```python
from build123d import *

# Parameters (mm, degrees)
BASE_FLANGE1_DEPTH = 6.35
SKETCH8_R          = 3.4
CUT_EXTRUDE1_DEPTH = 183.851914127
SKETCH9_R          = 34
CUT_EXTRUDE2_DEPTH = 183.851914127
SKETCH10_R         = 2.75
CUT_EXTRUDE3_DEPTH = 183.851914127


# Sheet-metal steps are written as plain solids
with BuildPart() as part:
    # Sketch2 → Base-Flange1 (new body)
    with BuildSketch(Plane(origin=(0, 0, 0), x_dir=(1, 0, 0), z_dir=(0, 1, 0))):
        with BuildLine():
            Line((0, 0), (50.76093065, 0))
            Line((50.76093065, 0), (107.880465325, 57.119534675))
            ThreePointArc((107.880465325, 57.119534675), (111.537953618, 118.761570635), (50.76093065, 129.682710556))
            Line((50.76093065, 129.682710556), (0, 90))
            Line((0, 90), (0, 0))
        make_face()
    extrude(amount=-BASE_FLANGE1_DEPTH)

    # Sketch8 → Cut-Extrude1 (cut, through all)
    with BuildSketch(Plane(origin=(0, 0, 0), x_dir=(1, 0, 0), z_dir=(0, 1, 0))):
        with Locations(Location((12.5, 79, 0), (0, 0, 270))):
            Circle(SKETCH8_R)
        with Locations(Location((12.5, 11, 0), (0, 0, 90))):
            Circle(SKETCH8_R)
    extrude(amount=-CUT_EXTRUDE1_DEPTH, mode=Mode.SUBTRACT)

    # Sketch9 → Cut-Extrude2 (cut, through all)
    with BuildSketch(Plane(origin=(0, 0, 0), x_dir=(1, 0, 0), z_dir=(0, 1, 0))):
        with Locations(Location((75, 90, 0), (0, 0, 270))):
            Circle(SKETCH9_R)
    extrude(amount=-CUT_EXTRUDE2_DEPTH, mode=Mode.SUBTRACT)

    # Sketch10 → Cut-Extrude3 (cut, through all)
    with BuildSketch(Plane(origin=(0, 0, 0), x_dir=(1, 0, 0), z_dir=(0, 1, 0))):
        with Locations(Location((75, 131, 0), (0, 0, 270))):
            Circle(SKETCH10_R)
        with Locations(Location((103.991378029, 118.991378029, 0), (0, 0, 270))):
            Circle(SKETCH10_R)
        with Locations(Location((116, 90, 0), (0, 0, 270))):
            Circle(SKETCH10_R)
        with Locations(Location((103.991378029, 61.008621971, 0), (0, 0, 270))):
            Circle(SKETCH10_R)
        with Locations(Location((75, 49, 0), (0, 0, 270))):
            Circle(SKETCH10_R)
        with Locations(Location((46.008621971, 61.008621971, 0), (0, 0, 270))):
            Circle(SKETCH10_R)
        with Locations(Location((34, 90, 0), (0, 0, 270))):
            Circle(SKETCH10_R)
        with Locations(Location((46.008621971, 118.991378029, 0), (0, 0, 270))):
            Circle(SKETCH10_R)
    extrude(amount=-CUT_EXTRUDE3_DEPTH, mode=Mode.SUBTRACT)


solid = part.part
```
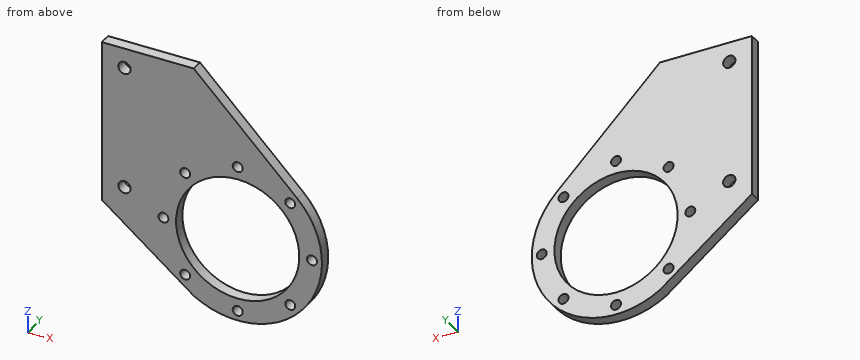
Input: part model. Units: mm. Frame: model coordinates. Coordinates: 2 decimals unless noted, no trailing zeros. Write each loop counter-clockwise with the first axis right and the second up, starting at its lowest first coordinate (ties: lowest second). Pieces come first, ordered by that corner, then holes. Notation, with made-up numbers: (8, 73.25) - (57, 73.25) arc R34 ccw to (57, 104.25) - close; hole circle Ø2 at (-18.75, 79). An arc over 180 degrees is marked (long way). Put each result on its own line as item: value. Start each with the question number.
1) Cut plane A-A (z = -12). Return the cut outline in (x, y), plus the area to 3 significant figures.
2) Cut plane B-B (x = 34). Return the cut outline in (y, z).
3) Cut plane C-C (y = -5.25). State how many separate pieces and enclosed holes the cut face has, plus the area to 3 significant figures.
4) Cut plane D-D (z = -79). Return the cut outline in (x, y).
5) Ray query, L1, parallel to X at y = -3.25, z = -90; L2, parallel to Z at x = 74, y = -1.75; L3, parallel to Z at x = 72.5, y = -2.5. Return the intervals inside material, ascending.
Resolved:
1. outline: (0, -6.35) - (9.25, -6.35) - (9.25, 0) - (0, 0) - close; (15.75, -6.35) - (62.76, -6.35) - (62.76, 0) - (15.75, 0) - close
1. area: 357 mm2
2. outline: (-6.35, -116.58) - (0, -116.58) - (0, -92.75) - (-6.35, -92.75) - close; (-6.35, -87.25) - (0, -87.25) - (0, 0) - (-6.35, 0) - close
3. separate pieces: 1
3. enclosed holes: 11
3. area: 8,270 mm2
4. outline: (0, -6.35) - (9.1, -6.35) - (9.1, 0) - (0, 0) - close; (15.9, -6.35) - (42.83, -6.35) - (42.83, 0) - (15.9, 0) - close; (107.17, -6.35) - (120.18, -6.35) - (120.18, 0) - (107.17, 0) - close
5. L1: x = 0 to 31.25, 36.75 to 41, 109 to 113.25, 118.75 to 121.5
5. L2: z = -136.49 to -133.56, -128.44 to -123.99, -56.01 to -51.56, -46.44 to -23.24
5. L3: z = -136.43 to -132.15, -129.85 to -123.91, -56.09 to -50.15, -47.85 to -21.74
